For this review, take the finished solid that the model builds, in its own axes (mm). Give positions to 0.01 mm unless a question says otherwise; leave off trailing zeros. Write each loop counter-clockwise with the first axis right and the second up, starting at its lowest first coordinate (ties: lowest second). Pieces come first, ordered by that corner, then holes. Notation, with made-up numbers: M -4,29 L 23,29 A24 ccw 23,50 Z; hole C -38,56 d4. An arc over 180 degrees is marked long. One line per item, written item: value. Start each with the question number.
Item 1: Clearance check with a flat-ended pin moving along its axis: pin 1 Ø1.5 at (x, y) = (84, 9.5) entering from +Z. State where the tip first meets the part, or that it passes through.
Item 2: Consider section A-A, the plane y = 9.25. Write out the cut boundary in (x, z), and give its area (3 significant figures).
Item 3: To check wall thickness, follow probe 1 along Y at (x, z) = (102.5, 20.25); probe 2 along X at (y, z) = (9, 15); probe 3 along Z at (x, y) = (85, 6.5). State the ranges of each line that lie inside material, in increasing order.
```python
from build123d import *

# Parameters (mm, degrees)
BOX023_W             = 30
BOX023_H             = 10
BOX023_DEPTH         = 11.5
CHAMFER019_1_SIZE2   = 8
CHAMFER019_1_SIZE    = 10
CHAMFER019_2_SIZE2   = 8
CHAMFER019_2_SIZE    = 10
FILLET002008005015_R = 4
FILLET002008005016_R = 1


with BuildPart() as part:
    # Box023 → Box023 (new body)
    with BuildSketch(Plane(origin=(80, 5, 3), x_dir=(1, 0, 0), z_dir=(0, 0, 1))):
        with Locations((15, 5)):
            Rectangle(BOX023_W, BOX023_H)
    extrude(amount=BOX023_DEPTH)

    # Chamfer019 1
    chamfer019_1_edges = [part.edges().sort_by_distance(p)[0] for p in [
        (110, 10, 14.5),
    ]]
    chamfer019_1_side = part.faces().sort_by_distance((110, 10, 8.75))[0]
    chamfer(chamfer019_1_edges, length=CHAMFER019_1_SIZE, length2=CHAMFER019_1_SIZE2, reference=chamfer019_1_side)

    # Chamfer019 2
    chamfer019_2_edges = [part.edges().sort_by_distance(p)[0] for p in [
        (80, 10, 14.5),
    ]]
    chamfer019_2_side = part.faces().sort_by_distance((80, 10, 8.75))[0]
    chamfer(chamfer019_2_edges, length=CHAMFER019_2_SIZE, length2=CHAMFER019_2_SIZE2, reference=chamfer019_2_side)

    # Fillet002008005015
    fillet002008005015_edges = [part.edges().sort_by_distance(p)[0] for p in [
        (88, 10, 14.5),
        (102, 10, 14.5),
    ]]
    fillet(fillet002008005015_edges, radius=FILLET002008005015_R)

    # Fillet002008005016
    fillet002008005016_edges = [part.edges().sort_by_distance(p)[0] for p in [
        (83.399512, 5, 8.74939),
        (88.189744, 5, 14.105213),
        (95, 5, 14.5),
        (101.810256, 5, 14.105213),
        (106.600488, 5, 8.74939),
        (83.399512, 15, 8.74939),
        (88.189744, 15, 14.105213),
        (95, 15, 14.5),
        (101.810256, 15, 14.105213),
        (106.600488, 15, 8.74939),
    ]]
    fillet(fillet002008005016_edges, radius=FILLET002008005016_R)


with BuildPart() as part_1:
    # Fillet002008005016 placement: moved
    add(part.part.moved(Location((0, 0, 7))))


solid = part_1.part
```
Model answer:
1. pin 1: stops at z = 17.44
2. outline: M 80,10 L 110,10 L 110,11.5 L 103.2,20 A4 ccw 100.08,21.5 L 89.92,21.5 A4 ccw 86.8,20 L 80,11.5 Z
2. area: 264 mm2
3. probe 1: y = 5.25 to 14.75
3. probe 2: x = 82.8 to 107.2
3. probe 3: z = 10 to 17.75
